Here's how the part is built. I have some questions about the finished solid (model axes, mm). A direction names the side the tool comes from. Coordinates: 2 decimals unless noted, no trailing zeros. Loops run counter-clockwise (first coordinate to the right, second up) from the corner with the lowest first, then second, coordinate; pieces in that order, holes last. Notation, with made-up numbers: M 66.25,63 L 96.25,63 A18 cw 96.25,78 Z; hole C -36,-27.5 d6. An arc over 180 degrees is marked long. Use one line per item in the form item = value. Start each with the question number.
(1) Will these pins go through, and if not, where does the flat tip stop? P1, Ø3, axis at y = 7, z = 9.5, coming from the +X side; P2, Ø3, axis at x = 16.75, y = 4.5, coming from the +Z side; P3, Ø1.5, axis at y = 7.5, z = 0.5, coming from the -X side (3 decimals); P4, Ø1.5, axis at x = -9, y = 5, coming from the +Z side.
(2) Imagine slicing it at B-B, the plane z = -2.5. Please give me the cut outline in (x, y), and give its area (3 significant figures).
(3) On a 3-axis mill with a long thin cutter (end or side, diameter ignored), from which of +Z, -Z, +X, -X, +Y, -Y can I reach the whole of each face in a straight line? I mean faces 1 (the cylindrical face through (17.14, 2.743, -10.528)), 2 (the flat face through (33.149, 4.437, 0.314)). Say none if no direction works.
(4) Imagine slicing it at A-A, the plane x = -16.75. Please give me the cut outline in (y, z), and give its area (3 significant figures).
(5) Imagine slicing it at D-D, the plane x = -38. Please give me the cut outline in (y, z), and give its area (3 significant figures).
(6) Thinking about a two-plate mould opening in X: for faces 3 (the flat face through (-33.11, 4.44, 0.28)), 4 (the flat face through (0, 9, -9)), 5 (the flat face through (-38.049, 4.437, -0.637)), which applies, +X half, -X half, draft (parallel to the pull), parting line (faces both ways), or undercut?
(7) Imagine slicing it at C-C, the plane y = 4.5. State how many separate pieces and enclosed holes the cut face has, and give its area (3 significant figures).
(8) Please list where these lines run through material, in increasing order: L1, parallel to Y at x = 16.75, z = -11.35; L2, parallel to X at y = 4.75, z = -10; L3, parallel to Z at x = 11.5, y = 3.
```python
from build123d import *

# Parameters (mm, degrees)
BOSS_EXTRUDE1_DEPTH  = 9
FILLET4_R            = 1
FILLET5_R            = 3
M3_CLEARANCE_HOLE1_D = 3.6


with BuildPart() as part:
    # Sketch1 → Boss-Extrude1 (new body)
    with BuildSketch(Plane(origin=(0, 0, 0), x_dir=(1, 0, 0), z_dir=(0, 1, 0))):
        Polygon((-25, 12.5), (-52.5, -12.5), (-41.5, -12.5), (-43.50199756, -9.725840963), (-23.453572501, 8.5), (23.453572501, 8.5), (44.071371219, -10.24345338), (41.5, -12.5), (52.5, -12.5), (25, 12.5), align=None)
    extrude(amount=BOSS_EXTRUDE1_DEPTH)

    # Fillet4
    fillet4_edges = [part.edges().sort_by_distance(p)[0] for p in [
        (52.5, 4.5, 12.5),
        (41.5, 4.5, 12.5),
        (-41.5, 4.5, 12.5),
        (-52.5, 4.5, 12.5),
    ]]
    fillet(fillet4_edges, radius=FILLET4_R)

    # Fillet5
    fillet5_edges = [part.edges().sort_by_distance(p)[0] for p in [
        (44.071371219, 4.5, 10.24345338),
        (25, 4.5, -12.5),
        (23.453572501, 4.5, -8.5),
        (-23.453572501, 4.5, -8.5),
        (-25, 4.5, -12.5),
        (-43.50199756, 4.5, 9.725840963),
    ]]
    fillet(fillet5_edges, radius=FILLET5_R)

    # M3 Clearance Hole1 (through all)
    with Locations(Plane.XY.offset(-8.5)):
        with Locations((-16.75, 4.5), (16.75, 4.5)):
            Hole(M3_CLEARANCE_HOLE1_D / 2)


solid = part.part
```
Answer:
q1.P1 = 50.78
q1.P2 = through
q1.P3 = -40.125
q1.P4 = -8.5
q2.outline = M -36,0 L -30.05,0 L -30.05,9 L -36,9 Z; M 30.05,0 L 36,0 L 36,9 L 30.05,9 Z
q2.area = 107 mm²
q3.face_1 = +Z, -Z
q3.face_2 = +Z, +Y, -Y
q4.outline = M 0,-12.5 L 2.7,-12.5 L 2.7,-8.5 L 0,-8.5 Z; M 6.3,-12.5 L 9,-12.5 L 9,-8.5 L 6.3,-8.5 Z
q4.area = 21.6 mm²
q5.outline = M 0,-0.68 L 9,-0.68 L 9,4.72 L 0,4.72 Z
q5.area = 48.7 mm²
q6.face_3 = undercut
q6.face_4 = draft
q6.face_5 = -X half
q7.separate_pieces = 3
q7.enclosed_holes = 0
q7.area = 448 mm²
q8.L1 = 0 to 2.7, 6.3 to 9
q8.L2 = -27.75 to -18.53, -14.97 to 14.97, 18.53 to 27.75
q8.L3 = -12.5 to -8.5
